Check sheet for the drawn part. Datum: minimum x, y, z corner. Units: mm. A direction names the side the tool comes from. Coordinates: 2 decimals unless noted, no trailing zeros. Order: outer loops, then holes, each group sorted by start corner. A loop starts at its lowest first (then second) coordinate and runs counter-clockwise, first axis right, second up. Notation, with made-up numbers: (44, -20) - (81, -20) arc R16 cw to (81, -3) - close; hole circle Ø3 at (-29, -9). An arc over 180 degrees is marked (long way). Return JSON: item names as keys, results as strings. Group by question number.
Item 1: Scan lines: probe 1 along X at (y, z) = (86, 17); probe 2 along X at (y, z) = (58, 18); probe 3 along Y at (x, z) = (113.5, 16.5) (3 decimals). Record each from-to range of solid material in increasing order.
Item 2: Draft check along Y on the marked faces 3 and 4. Enter one of: pulls with the +Y half, pulls with the -Y half, needs draft (parallel to the pull), parting line crosses it, or undercut.
Item 3: Gauge pin test, flat ends, axial feed: pin 1 (3 mm diameter, centred on x = 288.5, y = 80, fed in from +Z); pin 2 (1.5 mm diameter, centred on x = 189, y = 30.5, fed in from +Z) (3 decimals). Record the tip position at first contact, or that the pin passes through.
Item 4: Section check C-C on z = 7.25. Enter the section's corners in (x, y) (3 decimals), then the cut area to 3 significant figures.
Item 5: Tool access check on the marked faces 1 and 2. Record the directions out of +Z, -Z, +X, -X, +Y, -Y that give a thin tool (end or side, any length) a straight path to the whole face; none if there is none.
Item 6: Section check D-D on y = 26. Enter the section's corners in (x, z) (3 decimals).
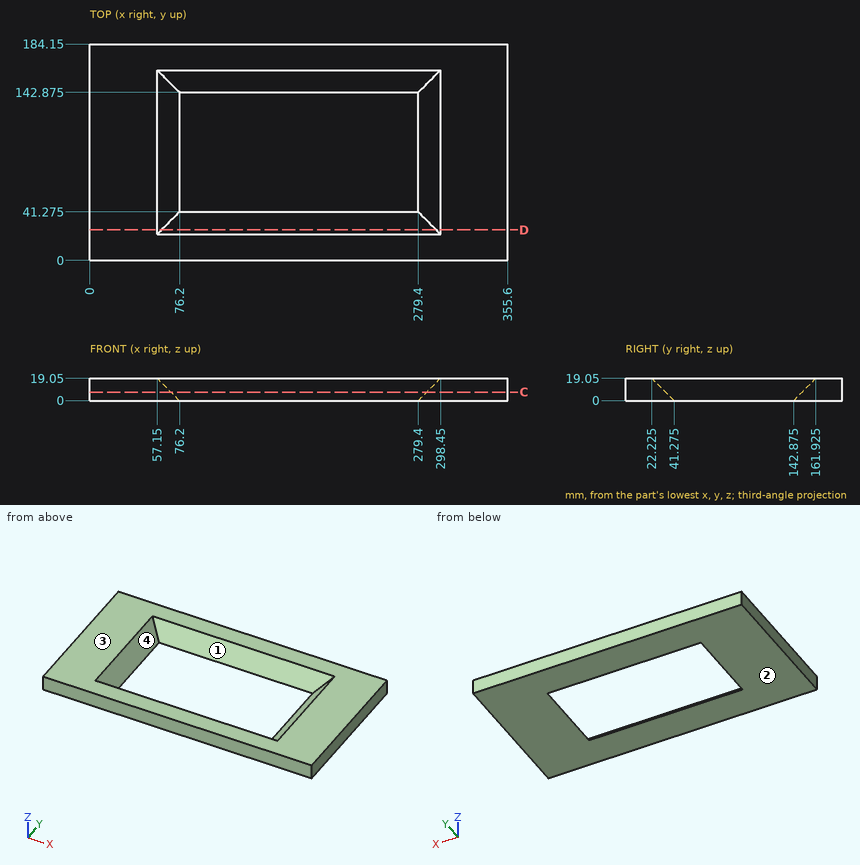
Computed:
{
 "1": {"probe 1": "x = 0 to 59.2, 296.4 to 355.6", "probe 2": "x = 0 to 58.2, 297.4 to 355.6", "probe 3": "y = 0 to 24.775, 159.375 to 184.15"},
 "2": {"face 3": "needs draft", "face 4": "undercut"},
 "3": {"pin 1": "stops at z = 10.6", "pin 2": "stops at z = 11.525"},
 "4": {"outline": "(0, 0) - (355.6, 0) - (355.6, 184.15) - (0, 184.15) - close; hole (68.95, 34.025) - (286.65, 34.025) - (286.65, 150.125) - (68.95, 150.125) - close", "area": "40,200 mm²"},
 "5": {"face 1": "+Z", "face 2": "-Z, +X, -X, +Y, -Y"},
 "6": {"outline": "(0, 0) - (355.6, 0) - (355.6, 19.05) - (298.45, 19.05) - (294.675, 15.275) - (60.925, 15.275) - (57.15, 19.05) - (0, 19.05) - close"}
}
